Autodesk Inventor part; units mm, degrees
ref_plane "YZ Plane" through (0, 0, 0) normal (1, 0, 0) x (0, 1, 0)
ref_plane "XZ Plane" through (0, 0, 0) normal (0, 1, 0) x (-1, 0, 0)
ref_plane "XY Plane" through (0, 0, 0) normal (0, 0, 1) x (1, 0, 0)
sketch "Sketch1" plane through (0, 0, 0) normal (0, 0, 1) x (1, 0, 0)
  circle A0 centre (32.4852, 19.5525) radius 11.1
  point P0 (0, 0)
extrude "Extrusion1" add sketch "Sketch1" along normal blind 7
sketch "Sketch7" plane through (32.4852, 19.5525, 7) normal (0, 0, 1) x (1, 0, 0)
  circle A0 centre (0, 0) radius 4.05
  circle A1 centre (0, 0) radius 11.1
  point P0 (-32.4852, -19.5525)
extrude "Extrusion7" cut sketch "Sketch7" against normal up to surface (7 mm away) contours A0
sketch "Sketch8" plane through (32.4852, 19.5525, 7) normal (0, 0, 1) x (1, 0, 0)
  circle A0 centre (0, 0) radius 4.05
  line L0 (4.05, 0) -> (5.8, 0)
  circle A1 centre (0, 0) radius 5.8
  circle A2 centre (0, 0) radius 11.1
  line L1 (11.1, 0) -> (9.35, 0)
  circle A3 centre (0, 0) radius 9.35
  point P0 (-32.4852, -19.5525)
  dimension "d18" = 1.75
  dimension "d19" = 1.75
extrude "Extrusion8" cut sketch "Sketch8" against normal blind 0.6 contours A3
sketch "Sketch9" plane through (32.4852, 19.5525, 0) normal (0, 0, -1) x (-1, 0, 0)
  circle A0 centre (0, 0) radius 5.8
  circle A1 centre (0, 0) radius 9.35
  point P0 (32.4852, -19.5525)
extrude "Extrusion9" cut sketch "Sketch9" against normal blind 0.6
properties part number "Metal bearing" material "Stainless Steel"
The listing builds one solid part. Answer for the finished solid, in the listing's coordinates (mm). A direction names the side the tool comes from. Coordinates: 2 decimals unless noted, no trailing zeros. Order: outer loops, then holes, each group sorted by start corner. A loop starts at its lowest first (then second) coordinate and runs counter-clockwise, first axis right, second up. Notation, with made-up numbers: (89, 79) -> (125, 79) arc R12 ccw to (125, 88) -> close; hole circle Ø5 at (15.25, -11.75). An arc over 180 degrees is marked (long way). Answer in a Markdown table with one row per item. Add a question column.
Item 1: Find section D-D (y = 21.5). Write down the section's boundary in (x, z), then the cut area to 3 significant figures.
Item 2: This flat-tipped pin is pushed along its axis until it touches: P1, Ø1.5, axis at y = 13.5, z = 6, coming from the -X side. Where does it stop, or does it pass through?
Item 3: Find the intervals of material crossed by L1, parallel to Z at x = 26, y = 23; L2, parallel to Y at x = 35, z = 5; L3, parallel to X at y = 20.75, z = 3.75, in increasing order. Write a range as from..to.
Item 4: Determine the mould class of faces 4 (the face through (34, 24, 7)), 5 (the face through (28, 24, 0.6)), 6 (the face through (42.74, 23.8, 3.45)) for opening direction Y: +Y half, -Y half, draft (parallel to the pull), parting line (faces both ways), or undercut.
Item 5: Find section A-A (y = 18). Write down the section's boundary in (x, z) (3 decimals).
Item 6: Find section C-C (x = 25.5). Write down the section's boundary in (y, z).
Item 7: Find section B-B (y = 10.75). Write down the section's boundary in (x, z), then the cut area to 3 significant figures.
Item 8: Which of the six approach directions +Z, -Z, +X, -X, +Y, -Y give full straight-line access (tool end or side, diameter ignored) to faces 1 (the face through (37, 24, 6.4)), 2 (the face through (28.17, 11.26, 0.3)), 3 (the face through (28, 11, 7))?
Result set:
| question | item | result |
|---|---|---|
| 1 | outline | (21.56, 0) -> (23.34, 0) -> (23.34, 0.6) -> (27.02, 0.6) -> (27.02, 0) -> (28.93, 0) -> (28.93, 7) -> (27.02, 7) -> (27.02, 6.4) -> (23.34, 6.4) -> (23.34, 7) -> (21.56, 7) -> close; (36.04, 0) -> (37.95, 0) -> (37.95, 0.6) -> (41.63, 0.6) -> (41.63, 0) -> (43.41, 0) -> (43.41, 7) -> (41.63, 7) -> (41.63, 6.4) -> (37.95, 6.4) -> (37.95, 7) -> (36.04, 7) -> close |
| 1 | area | 94.4 mm² |
| 2 | P1 | stops at x = 22.73 |
| 3 | L1 | z = 0.6..6.4 |
| 3 | L2 | y = 8.74..16.38, 22.73..30.36 |
| 3 | L3 | x = 21.45..28.62, 36.35..43.52 |
| 4 | face 4 | draft |
| 4 | face 5 | undercut |
| 4 | face 6 | parting line |
| 5 | outline | (21.494, 0) -> (23.265, 0) -> (23.265, 0.6) -> (26.897, 0.6) -> (26.897, 0) -> (28.745, 0) -> (28.745, 7) -> (26.897, 7) -> (26.897, 6.4) -> (23.265, 6.4) -> (23.265, 7) -> (21.494, 7) -> close; (36.226, 0) -> (38.074, 0) -> (38.074, 0.6) -> (41.705, 0.6) -> (41.705, 0) -> (43.476, 0) -> (43.476, 7) -> (41.705, 7) -> (41.705, 6.4) -> (38.074, 6.4) -> (38.074, 7) -> (36.226, 7) -> close |
| 6 | outline | (10.93, 0) -> (13.34, 0) -> (13.34, 0.6) -> (25.77, 0.6) -> (25.77, 0) -> (28.18, 0) -> (28.18, 7) -> (25.77, 7) -> (25.77, 6.4) -> (13.34, 6.4) -> (13.34, 7) -> (10.93, 7) -> close |
| 7 | outline | (25.72, 0) -> (29.33, 0) -> (29.33, 0.6) -> (35.64, 0.6) -> (35.64, 0) -> (39.25, 0) -> (39.25, 7) -> (35.64, 7) -> (35.64, 6.4) -> (29.33, 6.4) -> (29.33, 7) -> (25.72, 7) -> close |
| 7 | area | 87.1 mm² |
| 8 | face 1 | +Z |
| 8 | face 2 | -Z |
| 8 | face 3 | +Z, +X, -X, +Y, -Y |
